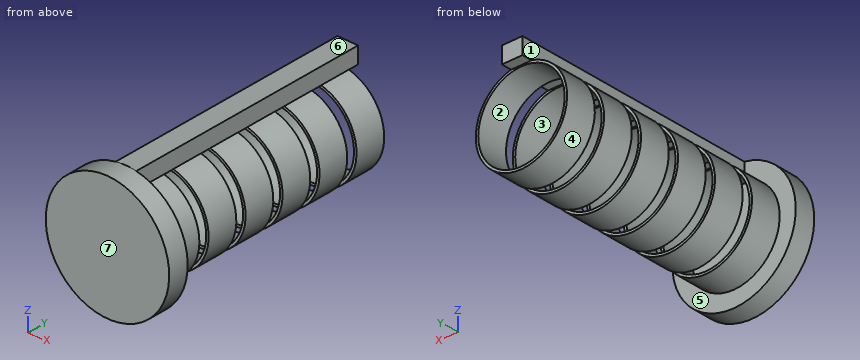
```python
from build123d import *

# Parameters (mm, degrees)
SKETCH2_R           = 38.1
BOSS_EXTRUDE1_DEPTH = 12.7
SKETCH3_W           = 12.7
SKETCH3_H           = 10.16
BOSS_EXTRUDE2_DEPTH = 152.4
SKETCH4_R           = 28.194
SKETCH4_R_2         = 26.67
LPATTERN1_COUNT     = 6
LPATTERN1_PITCH     = 25.4


with BuildPart() as part:
    # Sketch2 → Boss-Extrude1 (new body)
    with BuildSketch(Plane(origin=(0, 0, 0), x_dir=(1, 0, 0), z_dir=(0, 1, 0))):
        with Locations(Location((0, 0, 0), (0, 0, 270))):
            Circle(SKETCH2_R)
    extrude(amount=BOSS_EXTRUDE1_DEPTH)

    # Sketch3 → Boss-Extrude2 (add)
    with BuildSketch(Plane(origin=(0, 12.7, 0), x_dir=(1, 0, 0), z_dir=(0, 1, 0))):
        with Locations((0, -32.487106623)):
            Rectangle(SKETCH3_W, SKETCH3_H)
    extrude(amount=BOSS_EXTRUDE2_DEPTH)

    # Sweep-Thin1: sweep along a path in Sketch5
    with BuildLine(Plane.XY) as sweep_thin1_path:
        Line((0, 12.7), (0, 31.75))
    # Sketch4 → Sweep-Thin1 (sweep)
    with BuildSketch(Plane(origin=(0, 12.7, 0), x_dir=(1, 0, 0), z_dir=(0, 1, 0))):
        Circle(SKETCH4_R)
        Circle(SKETCH4_R_2, mode=Mode.SUBTRACT)
    sweep_thin1 = sweep(path=sweep_thin1_path.line)

    # LPattern1: Sweep-Thin1 ×6
    with Locations(*[(0, i * LPATTERN1_PITCH, 0) for i in range(1, LPATTERN1_COUNT)]):
        add(sweep_thin1)


solid = part.part
```
Here's how the part is built. I have some questions about the finished solid (model axes, mm). Face numbers are marked on the shaded views. A direction names the side the tool comes from. Give positions to 0.01 mm unless a question says otherwise; leave off trailing zeros. Write each loop counter-clockwise with the first axis right and the second up, starting at its lowest first coordinate (ties: lowest second). Pieces come first, ordered by that corner, then holes.
(1) If I drill on L1, parallel to Y at x = 22, z = 16; L2, parallel to X at y = 42, z = 0; L3, parallel to Y at x = -10, z = 21, over which ranges is the centre line in solid material (lowest first)?
Output values:
L1: y = 0 to 31.75, 38.1 to 57.15, 63.5 to 82.55, 88.9 to 107.95, 114.3 to 133.35, 139.7 to 158.75
L2: x = -28.19 to -26.67, 26.67 to 28.19
L3: y = 0 to 12.7
(2) Imagine slicing it at A-A, the plane x = 0. Count the separate pieces of the cut face and the enclosed holes in it, and give its area (3 significant figures).
Output values:
separate pieces: 6
enclosed holes: 0
area: 2,770 mm2
(3) Will these pins go through, and if not, where does the flat tip stop? pin 1 (3 mm diameter, centred on x = 4, y = 134.5, fed in from -Z); pin 2 (3 mm diameter, centred on x = -24, y = 28, fed in from -Z); pin 3 (10 mm diameter, centred on y = 94.5, z = -13, fed in from -X).
Output values:
pin 1: stops at z = -28.03
pin 2: stops at z = -16.99
pin 3: stops at x = -27.04
(4) Thinking about a two-plate mould opening in X: for the marked faces 1, 2, 3 and 4, which applies, pulls with the +X half, pulls with the -X half, needs draft (parallel to the pull), parting line crosses it, or undercut?
Output values:
face 1: pulls with the -X half
face 2: undercut
face 3: undercut
face 4: parting line crosses it
(5) Imagine slicing it at B-B, the plane y = 51.5. Write out the boundary of the cut face in (x, z).
Output values:
outline: (-6.35, 27.47) arc R28.19 ccw (long way) to (6.35, 27.47) - (6.35, 37.57) - (-6.35, 37.57) - close; hole circle Ø53.34 at (0, 0)
(6) On a 3-axis mill with a long thin cutter (end or side, diameter ignored), from which of +Z, -Z, +X, -X, +Y, -Y can I reach the whole of each face in a straight line? I mean the marked faces 5, 6 and 7. Say none if no direction works.
Output values:
face 5: +Y
face 6: +Z, +X, -X, +Y
face 7: +Z, -Z, +X, -X, -Y
